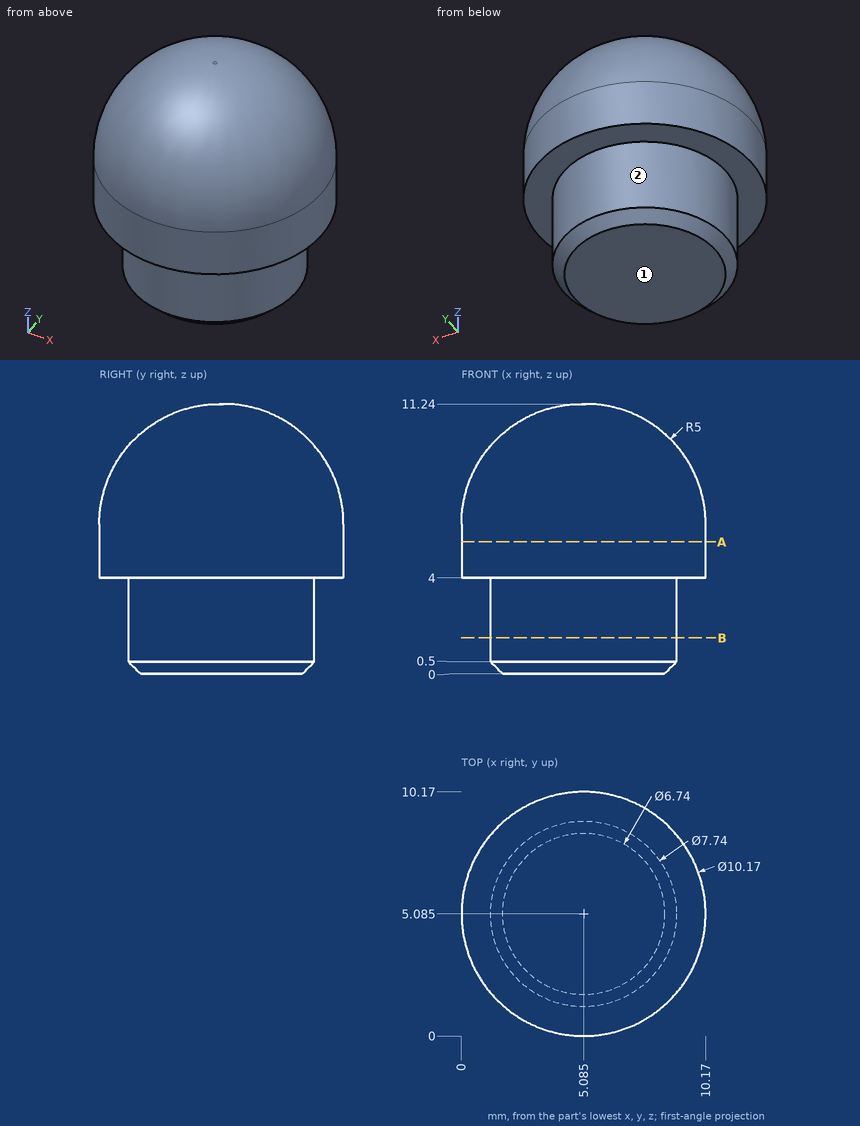
Can you work these out from the drawing? Everything is in mm from the part's minimum corner. A direction names the side the tool comes from. Coordinates: 2 decimals unless noted, no trailing zeros. Order: outer loops, then holes, each group sorted by start corner. A loop starts at its lowest first (then second) coordinate and runs counter-clockwise, first axis right, second up. Notation, with made-up numbers: (-6, 33.25) -> (43, 33.25) arc R21 cw to (43, 68.25) -> close; hole circle Ø3 at (64, -10.5). An arc over 180 degrees is marked (long way). Return JSON: item names as keys, results as strings.
1) I'm going to push flat-ended pins straight in: P1, Ø5, axis at x = 7.5, z = 2, coming from the +Y side; P2, Ø3, axis at x = 4.5, z = 9.5, coming from the -Y side. Where does each tip first touch, or does it pass through?
Conclusion:
{"P1": "stops at y = 10.09", "P2": "stops at y = 0.34"}
2) If we section it at A-A on z = 5.5: List the corners of the cut face in (x, y) for me (3 decimals), plus the area to 3 significant figures.
Conclusion:
{"outline": "circle Ø10.17 at (5.085, 5.085)", "area": "81.2 mm²"}
3) If we section it at B-B on z = 1.5: List the corners of the cut face in (x, y) for me (3 decimals), plus the area to 3 significant figures.
Conclusion:
{"outline": "circle Ø7.74 at (5.085, 5.085)", "area": "47.1 mm²"}
4) On a 3-axis mill with a long thin cutter (end or side, diameter ignored), from which of +Z, -Z, +X, -X, +Y, -Y can I reach the whole of each face in a straight line? I mean the marked faces 1 and 2. Say none if no direction works.
Conclusion:
{"face 1": "-Z, +X, -X, +Y, -Y", "face 2": "-Z"}
5) If I drill on probe 1 along Y at (x, z) = (5, 9.5); probe 2 along Z at (x, y) = (3.25, 2.5); probe 3 along Z at (x, y) = (0.5, 5), over which ranges is the centre line in solid material (lowest first)?
Conclusion:
{"probe 1": "y = 1.21 to 8.96", "probe 2": "z = 0 to 10.17", "probe 3": "z = 4 to 8.42"}
